```python
from build123d import *

# Parameters (mm, degrees)
SKETCH1_W                      = 260.35
SKETCH1_H                      = 63.5
BASE_FLANGE1_DEPTH             = 3.2639
EDGE_FLANGE1_STRIP_W           = 18.36928
EDGE_FLANGE1_STRIP_H           = 3.2639
EDGE_FLANGE1_STRIP_CUT_DEPTH   = 63.5
EDGE_FLANGE1_STRIP_2_W         = 18.36928
EDGE_FLANGE1_STRIP_2_H         = 3.2639
EDGE_FLANGE1_STRIP_CUT_2_DEPTH = 63.5
EDGE_FLANGE1_DEPTH             = 63.5
EDGE_FLANGE1_BEND_DEPTH        = 63.5
F_10_0_1935_DIAMETER_HOLE1_D   = 4.9149
FILLET1_R                      = 1.27
F_1_4_CLEARANCE_HOLE1_D        = 6.7564


# Sheet-metal steps are written as plain solids
with BuildPart() as part:
    # Sketch1 → Base-Flange1 (new body)
    with BuildSketch(Plane.XY):
        Rectangle(SKETCH1_W, SKETCH1_H)
    extrude(amount=-BASE_FLANGE1_DEPTH)

    # Edge-Flange1 strip (across the edge) → Edge-Flange1 strip cut (cut)
    with BuildSketch(Plane(origin=(130.175, 31.75, -3.2639), x_dir=(-1, 0, 0), z_dir=(0, -1, 0))):
        with Locations((-3.2639, -1.63195)):
            Rectangle(EDGE_FLANGE1_STRIP_W, EDGE_FLANGE1_STRIP_H)
    extrude(amount=EDGE_FLANGE1_STRIP_CUT_DEPTH, mode=Mode.SUBTRACT)

    # Edge-Flange1 strip 2 (across the edge) → Edge-Flange1 strip cut 2 (cut)
    with BuildSketch(Plane(origin=(-130.175, -31.75, -3.2639), x_dir=(1, 0, 0), z_dir=(0, 1, 0))):
        with Locations((-3.2639, -1.63195)):
            Rectangle(EDGE_FLANGE1_STRIP_2_W, EDGE_FLANGE1_STRIP_2_H)
    extrude(amount=EDGE_FLANGE1_STRIP_CUT_2_DEPTH, mode=Mode.SUBTRACT)

    # Edge-Flange1 section (across the edge) → Edge-Flange1 (add)
    with BuildSketch(Plane(origin=(130.175, 31.75, -3.2639), x_dir=(-1, 0, 0), z_dir=(0, -1, 0))):
        with BuildLine():
            Line((0, 2.65684), (0, 15.7861))
            Line((0, 15.7861), (3.2639, 15.7861))
            Line((3.2639, 15.7861), (3.2639, 2.65684))
            ThreePointArc((3.2639, 2.65684), (4.042070419, 0.778170419), (5.92074, 0))
            Line((5.92074, 0), (5.92074, -3.2639))
            ThreePointArc((5.92074, -3.2639), (1.734144596, -1.529755404), (0, 2.65684))
        make_face()
    extrude(amount=EDGE_FLANGE1_DEPTH)

    # Edge-Flange1 section 2 (across the edge) → Edge-Flange1 bend (add)
    with BuildSketch(Plane(origin=(-130.175, -31.75, -3.2639), x_dir=(1, 0, 0), z_dir=(0, 1, 0))):
        with BuildLine():
            Line((0, 2.65684), (0, 15.7861))
            Line((0, 15.7861), (3.2639, 15.7861))
            Line((3.2639, 15.7861), (3.2639, 2.65684))
            ThreePointArc((3.2639, 2.65684), (4.042070419, 0.778170419), (5.92074, 0))
            Line((5.92074, 0), (5.92074, -3.2639))
            ThreePointArc((5.92074, -3.2639), (1.734144596, -1.529755404), (0, 2.65684))
        make_face()
    extrude(amount=EDGE_FLANGE1_BEND_DEPTH)

    # #10 (0.1935) Diameter Hole1 (through all)
    with Locations(Plane(origin=(130.175, 0, 0), x_dir=(0, 0, -1), z_dir=(1, 0, 0))):
        with Locations((12.7, 22.225), (12.7, -22.225)):
            Hole(F_10_0_1935_DIAMETER_HOLE1_D / 2)

    # Fillet1
    fillet1_edges = [part.edges().sort_by_distance(p)[0] for p in [
        (128.54305, 31.75, -19.05),
        (128.54305, -31.75, -19.05),
        (-128.54305, -31.75, -19.05),
        (-128.54305, 31.75, -19.05),
    ]]
    fillet(fillet1_edges, radius=FILLET1_R)

    # 1/4 Clearance Hole1 (through all)
    with Locations(Plane.XY):
        with Locations((-107.95, 0), (107.95, 0)):
            Hole(F_1_4_CLEARANCE_HOLE1_D / 2)


solid = part.part
```
Geometry check sheet. Reference: the model listing, model coordinates, mm. A direction names the side the tool comes from. Give positions to 0.01 mm unless a question says otherwise; leave off trailing zeros. Write each loop counter-clockwise with the first axis right and the second up, starting at its lowest first coordinate (ties: lowest second). Pieces come first, ordered by that corner, then holes.
1) Section check D-D, the plane y = 27.5. Record the boundary of the cut face in (x, z) (3 decimals).
2) Release check for a two-part mould opening along Z. For faces 3 (the cylindrical face through (-128.57, -23.72, -14.65)), 4 (the cylindrical face through (128.395, 0.444, -1.688)), 5 (the flat face through (-2, 0, -3.264)), 6 (the cylindrical face through (-111.071, -1.294, -1.655)) record: pulls with the +Z half, pulls with the -Z half, needs draft (parallel to the pull), parting line crosses it, or undercut.
3) Section check A-A, the plane x = 107.95. Record the boundary of the cut face in (y, z), and give its area (3 significant figures).
4) Gauge pin test, flat ends, axial feed: pin 1 (1 mm diameter, centred on y = 5, z = -2.5, fed in from -X); pin 2 (5 mm diameter, centred on x = 96.5, y = -5, fed in from -Z). Record the tip position at first contact, or that the pin passes through.
5) Section check B-B, the plane y = 0. Record the boundary of the cut face in (x, z) (3 decimals).
6) Section check C-C, the plane z = -12.7. Record the boundary of the cut face in (x, y) (3 decimals), and give its area (3 significant figures).
7) Access from +Z, -Z, +X, -X, +Y, -Y to the whole of each face (thin tool, end or side, straight path). Record for faces 1 (the flat face through (-2, 0, 0)), 2 (the flat face through (126.911, 0, -13)).
8) Material ranges on L1, parallel to Y at x = -129.45, z = -12.7; L2, parallel to Y at x = -107.95, z = -0.9; L3, parallel to X at y = 3, z = -1, recorded low to high.
Computed:
1. outline: (-130.175, -19.05) - (-126.911, -19.05) - (-126.911, -5.921) arc R2.657 cw to (-124.254, -3.264) - (124.254, -3.264) arc R2.657 cw to (126.911, -5.921) - (126.911, -19.05) - (130.175, -19.05) - (130.175, -5.921) arc R5.921 ccw to (124.254, 0) - (-124.254, 0) arc R5.921 ccw to (-130.175, -5.921) - close
2. face 3: undercut
2. face 4: pulls with the +Z half
2. face 5: pulls with the -Z half
2. face 6: needs draft
3. outline: (-31.75, -3.26) - (-3.38, -3.26) - (-3.38, 0) - (-31.75, 0) - close; (3.38, -3.26) - (31.75, -3.26) - (31.75, 0) - (3.38, 0) - close
3. area: 185 mm2
4. pin 1: stops at x = -129.4
4. pin 2: stops at z = -3.26
5. outline: (-130.175, -19.05) - (-126.911, -19.05) - (-126.911, -5.921) arc R2.657 cw to (-124.254, -3.264) - (-111.328, -3.264) - (-111.328, 0) - (-124.254, 0) arc R5.921 ccw to (-130.175, -5.921) - close; (-104.572, -3.264) - (104.572, -3.264) - (104.572, 0) - (-104.572, 0) - close; (111.328, -3.264) - (124.254, -3.264) arc R2.657 cw to (126.911, -5.921) - (126.911, -19.05) - (130.175, -19.05) - (130.175, -5.921) arc R5.921 ccw to (124.254, 0) - (111.328, 0) - close
6. outline: (-130.175, -31.75) - (-126.911, -31.75) - (-126.911, -24.682) - (-130.175, -24.682) - close; (-130.175, -19.768) - (-126.911, -19.768) - (-126.911, 19.768) - (-130.175, 19.768) - close; (-130.175, 24.682) - (-126.911, 24.682) - (-126.911, 31.75) - (-130.175, 31.75) - close; (126.911, -31.75) - (130.175, -31.75) - (130.175, -24.682) - (126.911, -24.682) - close; (126.911, -19.768) - (130.175, -19.768) - (130.175, 19.768) - (126.911, 19.768) - close; (126.911, 24.682) - (130.175, 24.682) - (130.175, 31.75) - (126.911, 31.75) - close
6. area: 350 mm2
7. face 1: +Z, +X, -X, +Y, -Y
7. face 2: -Z, +Y, -Y
8. L1: y = -31.75 to -24.68, -19.77 to 19.77, 24.68 to 31.75
8. L2: y = -31.75 to -3.38, 3.38 to 31.75
8. L3: x = -127.55 to -109.5, -106.4 to 106.4, 109.5 to 127.55
